Here's how the part is built. I have some questions about the finished solid (model axes, mm). Face numbers are marked on the shaded views. A direction names the side the tool comes from. Coordinates: 2 decimals unless noted, no trailing zeros. Write each loop counter-clockwise with the first axis right and the second up, starting at its lowest first coordinate (ties: lowest second). Pieces come first, ordered by that corner, then holes.
Item 1: If I drill on line 1 (X direction, y = 10, z = -36); line 2 (X direction, y = 1.25, z = -40.5); line 3 (Z direction, x = 37.5, y = 10.25), over which ranges is the centre line in solid material (lowest first)?
Item 2: If we section it at C-C (x = 16): Please give me the cut outline in (y, z).
Item 3: If we section it at D-D (x = 37): Please give me the cut outline in (y, z).
Item 4: If we section it at A-A (x = 0): Please give me the cut outline in (y, z), then the cut area to 3 significant figures.
Item 5: For the marked faces 1, 2 and 3, which set-ups out of +Z, -Z, +X, -X, +Y, -Y let a thin tool reach every point of the face, with its end or its side?
Item 6: If we section it at B-B (z = 57.5): Please give me the cut outline in (x, y), then the cut area to 3 significant figures.
Item 7: I'm going to push flat-ended pins straight in: pin 1 Ø2 at (y, z) = (7, -2) entering from -X; pin 2 Ø0.6 at (x, y) = (61.5, 9.5) entering from -Z; pin 3 Ø5 at (x, y) = (7, 9) entering from -Z. Where does each tip first touch, or does it pass through?
Item 8: We'd pull the mould along X, two halves only. Please class the marked faces 4, 5 and 6: +X half, -X half, draft (parallel to the pull), parting line (faces both ways), or undercut.
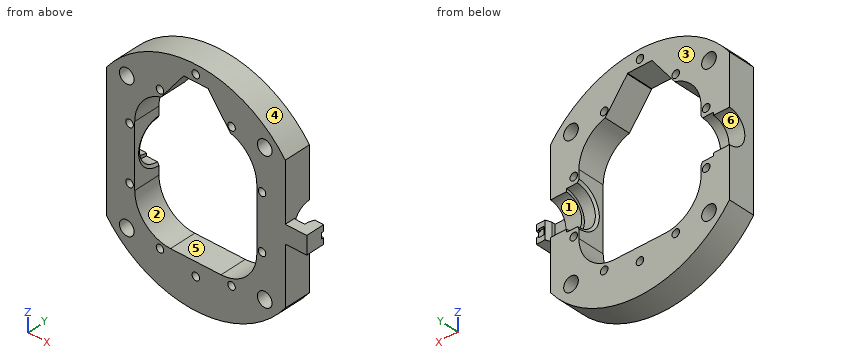
from build123d import *
from OCP.BRepFilletAPI import BRepFilletAPI_MakeChamfer

# Parameters (mm, degrees)
SKETCH2_R               = 62.5
SKETCH2_W               = 68.2
SKETCH2_H               = 75
BOSS_EXTRUDE1_DEPTH     = 15
SKETCH7_W               = 7
SKETCH7_H               = 11.1
CUT_EXTRUDE1_DEPTH      = 122.918866465
CUT_EXTRUDE1_DEPTH_BACK = 122.918866465
SKETCH8_R               = 9.5
FILLET1_R               = 20
SKETCH9_R               = 2.1
CUT_EXTRUDE2_DEPTH      = 90.652105542
CHAMFER1_SIZE           = 1.5
CHAMFER1_SIZE2          = 0.866025404
SKETCH10_R              = 4.1
CUT_EXTRUDE3_DEPTH      = 90.652105542
CUT_EXTRUDE4_DEPTH      = 90.652105542
SKETCH12_W              = 10
SKETCH12_H              = 5.5
BOSS_EXTRUDE2_DEPTH     = 12
BOSS_EXTRUDE3_START     = 6
SKETCH14_W              = 10
SKETCH14_H              = 3.7
BOSS_EXTRUDE3_DEPTH     = 6
BOSS_EXTRUDE4_DEPTH     = 1.3
CHAMFER2_SIZE           = 3
CHAMFER2_SIZE2          = 1.091910703
SKETCH16_W              = 14
SKETCH16_H              = 16
CUT_EXTRUDE5_DEPTH      = 90.652105542
CHAMFER3_DEPTH          = 15
CUT_EXTRUDE6_DEPTH      = 90.652105542


with BuildPart() as part:
    # Sketch2 → Boss-Extrude1 (new body)
    with BuildSketch(Plane(origin=(0, 0, 0), x_dir=(1, 0, 0), z_dir=(0, 1, 0))):
        with Locations(Location((0, 0, 0), (0, 0, 270))):
            Circle(SKETCH2_R)
        Rectangle(SKETCH2_W, SKETCH2_H, mode=Mode.SUBTRACT)
    extrude(amount=BOSS_EXTRUDE1_DEPTH)

    # Sketch7 → Cut-Revolve2 (revolve, cut)
    with BuildSketch(Plane(origin=(0, 15, 0), x_dir=(1, 0, 0), z_dir=(0, 1, 0))):
        with Locations((-37.6, 5.55)):
            Rectangle(SKETCH7_W, SKETCH7_H)
        with Locations((37.6, 5.55)):
            Rectangle(SKETCH7_W, SKETCH7_H)
    revolve(axis=Axis((62.5, 15, 0), (-1, 0, 0)), mode=Mode.SUBTRACT)

    # Sketch8 → Cut-Extrude1 (cut, two sides: drawn at the far end of the back side and taken through both)
    with BuildSketch(Plane.ZY.offset(-41.1).offset(-CUT_EXTRUDE1_DEPTH_BACK)):
        with Locations((0, 15)):
            Circle(SKETCH8_R)
    extrude(amount=CUT_EXTRUDE1_DEPTH + CUT_EXTRUDE1_DEPTH_BACK, mode=Mode.SUBTRACT)

    # Fillet1
    fillet1_edges = [part.edges().sort_by_distance(p)[0] for p in [
        (-34.1, 7.5, -37.5),
        (-34.1, 7.5, 37.5),
        (34.1, 7.5, 37.5),
        (34.1, 7.5, -37.5),
    ]]
    fillet(fillet1_edges, radius=FILLET1_R)

    # Sketch9 → Cut-Extrude2 (cut, through all)
    with BuildSketch(Plane(origin=(0, 15, 0), x_dir=(1, 0, 0), z_dir=(0, 1, 0))):
        with Locations(Location((-37, 15.198684154, 0), (0, 0, 270))):
            Circle(SKETCH9_R)
        with Locations(Location((37, 15.198684154, 0), (0, 0, 270))):
            Circle(SKETCH9_R)
        with Locations(Location((37, -15.198684154, 0), (0, 0, 270))):
            Circle(SKETCH9_R)
        with Locations(Location((-37, -15.198684154, 0), (0, 0, 270))):
            Circle(SKETCH9_R)
        with Locations(Location((-20, 40.311288741, 0), (0, 0, 270))):
            Circle(SKETCH9_R)
        with Locations(Location((20, 40.311288741, 0), (0, 0, 270))):
            Circle(SKETCH9_R)
        with Locations(Location((20, -40.311288741, 0), (0, 0, 270))):
            Circle(SKETCH9_R)
        with Locations(Location((-20, -40.311288741, 0), (0, 0, 270))):
            Circle(SKETCH9_R)
        with Locations(Location((0, 45, 0), (0, 0, 270))):
            Circle(SKETCH9_R)
        with Locations(Location((0, -57.5, 0), (0, 0, 270))):
            Circle(SKETCH9_R)
    extrude(amount=-CUT_EXTRUDE2_DEPTH, mode=Mode.SUBTRACT)

    # Chamfer1: one chamfer whose edges measure the first distance from different faces: ONE call of the kernel's chamfer builder (chamfer() names one face for all edges)
    chamfer1_edges_1 = [part.edges().sort_by_distance(p)[0] for p in [
        (-34.1, 3.9, 0),
    ]]
    chamfer1_side_1 = [part.faces().sort_by_distance(p)[0] for p in [
        (-34.1, 0.380788655, 0),
    ]]
    chamfer1_edges_2 = [part.edges().sort_by_distance(p)[0] for p in [
        (34.1, 3.9, 0),
    ]]
    chamfer1_side_2 = [part.faces().sort_by_distance(p)[0] for p in [
        (34.1, 0.380788655, 0),
    ]]
    chamfer1 = BRepFilletAPI_MakeChamfer(part.part.solid().wrapped)
    for e in chamfer1_edges_1:
        chamfer1.Add(CHAMFER1_SIZE, CHAMFER1_SIZE2, e.wrapped, chamfer1_side_1[0].wrapped)  # the first distance lies on this face
    for e in chamfer1_edges_2:
        chamfer1.Add(CHAMFER1_SIZE, CHAMFER1_SIZE2, e.wrapped, chamfer1_side_2[0].wrapped)  # the first distance lies on this face
    add(Compound.cast(chamfer1.Shape()), mode=Mode.REPLACE)

    # Sketch10 → Cut-Extrude3 (cut, through all)
    with BuildSketch(Plane.XZ):
        with Locations(Location((38.537319575, -38.537319575, 0), (0, 0, 270))):
            Circle(SKETCH10_R)
        with Locations(Location((-38.537319575, -38.537319575, 0), (0, 0, 270))):
            Circle(SKETCH10_R)
        with Locations(Location((-38.537319575, 38.537319575, 0), (0, 0, 270))):
            Circle(SKETCH10_R)
        with Locations(Location((38.537319575, 38.537319575, 0), (0, 0, 270))):
            Circle(SKETCH10_R)
    extrude(amount=-CUT_EXTRUDE3_DEPTH, mode=Mode.SUBTRACT)

    # Sketch11 → Cut-Extrude4 (cut, through all)
    with BuildSketch(Plane.XZ):
        with BuildLine():
            Line((50, -37.5), (50, 37.5))
            ThreePointArc((50, 37.5), (62.5, 0), (50, -37.5))
        make_face()
    extrude(amount=-CUT_EXTRUDE4_DEPTH, mode=Mode.SUBTRACT)

    # Sketch12 → Boss-Extrude2 (add)
    with BuildSketch(Plane(origin=(50, 0, 0), x_dir=(0, 0, -1), z_dir=(1, 0, 0))):
        with Locations((0, 2.75)):
            Rectangle(SKETCH12_W, SKETCH12_H)
    extrude(amount=BOSS_EXTRUDE2_DEPTH)

    # Sketch14 → Boss-Extrude3 (add)
    with BuildSketch(Plane(origin=(50, 0, 0), x_dir=(0, 0, -1), z_dir=(1, 0, 0)).offset(BOSS_EXTRUDE3_START)):
        with Locations((0, 7.35)):
            Rectangle(SKETCH14_W, SKETCH14_H)
    extrude(amount=BOSS_EXTRUDE3_DEPTH)

    # Sketch15 → Boss-Extrude4 (add)
    with BuildSketch(Plane(origin=(0, 9.2, 0), x_dir=(1, 0, 0), z_dir=(0, 1, 0))):
        Polygon((60.9, -2.2), (60.9, -1.6), (62, -1.6), (62, -5), (56, -5), (56, 5), (62, 5), (62, 1.6), (60.9, 1.6), (60.9, 2.2), (57.7, 2.2), (57.7, -2.2), align=None)
    extrude(amount=BOSS_EXTRUDE4_DEPTH)

    # Chamfer2
    chamfer2_edges = [part.edges().sort_by_distance(p)[0] for p in [
        (56, 10.5, 0),
    ]]
    chamfer2_side = [part.faces().sort_by_distance(p)[0] for p in [
        (56, 8, 0),
    ]]
    chamfer(chamfer2_edges, length=CHAMFER2_SIZE, length2=CHAMFER2_SIZE2, reference=chamfer2_side[0])

    # Sketch16 → Cut-Extrude5 (cut, through all)
    with BuildSketch(Plane.XZ):
        with Locations((0, 45.5)):
            Rectangle(SKETCH16_W, SKETCH16_H)
    extrude(amount=-CUT_EXTRUDE5_DEPTH, mode=Mode.SUBTRACT)

    # Chamfer3: read off the stored shape, not the designer's step
    # Chamfer3 outline → Chamfer3 (cut)
    with BuildSketch(Plane(origin=(0, 0, 0), x_dir=(1, 0, 0), z_dir=(0, 1, 0))):
        with BuildLine():
            Line((7, -53.150946691), (19.451351351, -36.770781996))
            ThreePointArc((19.451351351, -36.770781996), (16.800403682, -37.316856965), (14.1, -37.5))
            Line((14.1, -37.5), (7, -37.5))
            Line((7, -37.5), (7, -53.150946691))
        make_face()
        with BuildLine():
            ThreePointArc((-14.1, -37.5), (-16.800403682, -37.316856965), (-19.451351351, -36.770781996))
            Line((-19.451351351, -36.770781996), (-7, -53.150946691))
            Line((-7, -53.150946691), (-7, -37.5))
            Line((-7, -37.5), (-14.1, -37.5))
        make_face()
    extrude(amount=CHAMFER3_DEPTH, mode=Mode.SUBTRACT)

    # Sketch18 → Cut-Extrude6 (cut, through all)
    with BuildSketch(Plane.XZ):
        with BuildLine():
            Line((-50, 37.5), (-50, -37.5))
            ThreePointArc((-50, -37.5), (-62.5, 0), (-50, 37.5))
        make_face()
    extrude(amount=-CUT_EXTRUDE6_DEPTH, mode=Mode.SUBTRACT)


solid = part.part
Answer list:
1. line 1: x = -50 to -41.76, -35.32 to -21.7, 21.7 to 35.32, 41.76 to 50
1. line 2: x = -47.6 to -42.14, -34.94 to -22.09, -17.91 to 17.91, 22.09 to 34.94, 42.14 to 47.6
1. line 3: z = -50 to -42.5, -34.57 to -17.24, -13.16 to -10.03, 10.03 to 13.16, 17.24 to 34.57, 42.5 to 50
2. outline: (0, -60.42) - (15, -60.42) - (15, -37.41) - (0, -37.41) - close; (0, 41.31) - (15, 41.31) - (15, 60.42) - (0, 60.42) - close
3. outline: (0, -50.37) - (15, -50.37) - (15, -42.34) - (0, -42.34) - close; (0, -34.74) - (15, -34.74) - (15, -17.3) - (0, -17.3) - close; (0, -13.1) - (15, -13.1) - (15, -11.1) arc R11.1 cw to (15, 11.1) - (15, 13.1) - (0, 13.1) - close; (0, 17.3) - (15, 17.3) - (15, 34.74) - (0, 34.74) - close; (0, 42.34) - (15, 42.34) - (15, 50.37) - (0, 50.37) - close
4. outline: (0, -62.5) - (15, -62.5) - (15, -47.1) - (0, -47.1) - close; (0, -42.9) - (15, -42.9) - (15, -37.5) - (0, -37.5) - close; (0, 53.5) - (15, 53.5) - (15, 55.4) - (0, 55.4) - close; (0, 59.6) - (15, 59.6) - (15, 62.5) - (0, 62.5) - close
4. area: 384 mm2
5. face 1: -X, +Y
5. face 2: +Y, -Y
5. face 3: +Z, -Z, +X, -X, +Y
6. outline: (-24.49, 0) - (-2.1, 0) - (-2.1, 15) - (-24.49, 15) - close; (2.1, 0) - (24.49, 0) - (24.49, 15) - (2.1, 15) - close
6. area: 672 mm2
7. pin 1: stops at x = 56
7. pin 2: stops at z = -5
7. pin 3: stops at z = -62.34
8. face 4: parting line
8. face 5: undercut
8. face 6: draft
